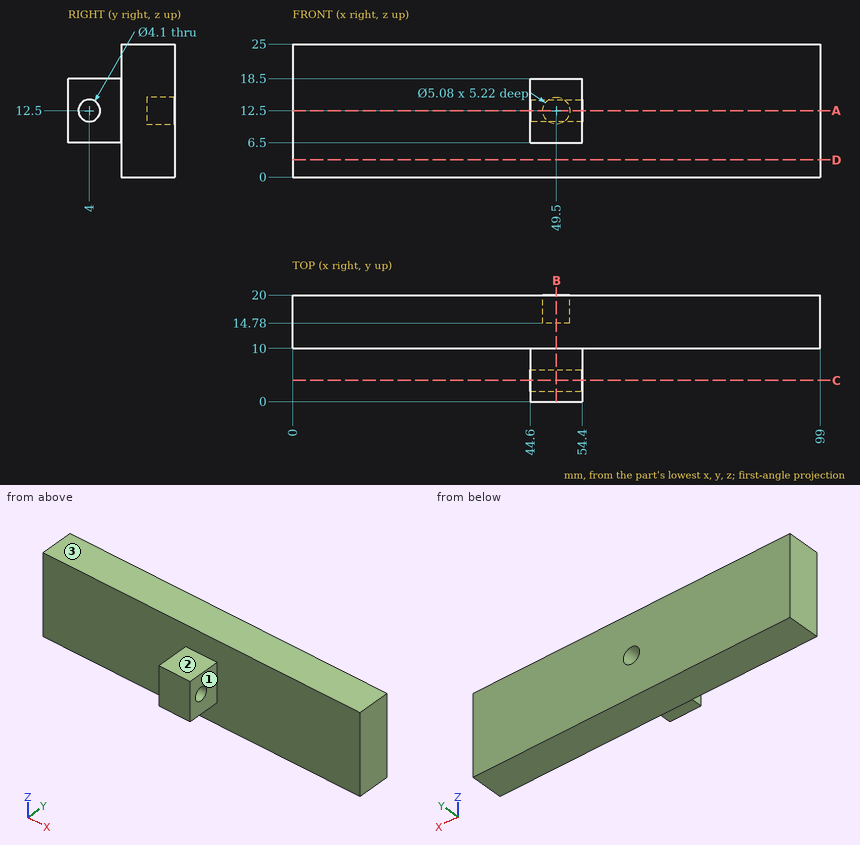
Part print with two shaded views. Sizes in mm from the minimum x, y, z corner. A direction names the side the tool comes from. Round coordinates to 2 decimals unless told otherwise and drop trailing zeros. Write each loop counter-clockwise with the first axis right and the second up, starting at its lowest first coordinate (ties: lowest second). Pieces come first, ordered by that corner, then holes. Notation, with made-up numbers: (5, -4.5) - (51, -4.5) arc R27 cw to (51, 21.5) - close; hole circle Ø2 at (82.25, 86.5). An arc over 180 degrees is marked (long way). Use CSV: the item, a comma, the result in double quotes.
Item 1: Slice it at D-D, the plane z = 3.25. Write the cut outline in (x, y), then the cut area to 3 significant figures.
Results list:
outline,"(0, 10) - (99, 10) - (99, 20) - (0, 20) - close"
area,"990 mm²"
Item 2: Tool access for the marked faces 1, 2 and 3: list every direction of +Z, -Z, +X, -X, +Y, -Y with a clear straight run to the whole face (end or side of a thin tool).
Results list:
face 1,"+Z, -Z, +X, -Y"
face 2,"+Z, +X, -X, -Y"
face 3,"+Z, +X, -X, +Y, -Y"
Item 3: Wall check: L1, parallel to Y at x = 52, z = 12.5; L2, parallel to X at y = 18.25, z = 12.5; L3, parallel to Y at x = 39, z = 15.25. Give the ranges that are in metal, low to high.
Results list:
L1,"y = 0 to 1.95, 6.05 to 14.78"
L2,"x = 0 to 46.96, 52.04 to 99"
L3,"y = 10 to 20"
Item 4: Slice it at A-A, the plane z = 12.5. Write the cut outline in (x, y).
Results list:
outline,"(0, 10) - (44.6, 10) - (44.6, 6.05) - (54.4, 6.05) - (54.4, 10) - (99, 10) - (99, 20) - (52.04, 20) - (52.04, 14.78) - (46.96, 14.78) - (46.96, 20) - (0, 20) - close; (44.6, 0) - (54.4, 0) - (54.4, 1.95) - (44.6, 1.95) - close"
Item 5: Slice it at C-C, the plane y = 4. Write the cut outline in (x, z), then the cut area to 3 significant figures.
Results list:
outline,"(44.6, 6.5) - (54.4, 6.5) - (54.4, 10.45) - (44.6, 10.45) - close; (44.6, 14.55) - (54.4, 14.55) - (54.4, 18.5) - (44.6, 18.5) - close"
area,"77.4 mm²"
Item 6: Flat gauge pins, fed straight in: P1, Ø3, axis at x = 49.5, z = 12.5, coming from the +Y side; P2, Ø11, axis at y = 2.5, z = 13.5, coming from the +X side; P3, Ø3, axis at x = 50, y = 6, coming from the -Z side. Where does each tip first touch, or does it go through?
Results list:
P1,"stops at y = 14.78"
P2,"stops at x = 54.4"
P3,"stops at z = 6.5"
Item 7: Slice it at B-B, the plane x = 49.5. Write the cut outline in (y, z).
Results list:
outline,"(0, 6.5) - (10, 6.5) - (10, 0) - (20, 0) - (20, 9.96) - (14.78, 9.96) - (14.78, 15.04) - (20, 15.04) - (20, 25) - (10, 25) - (10, 18.5) - (0, 18.5) - close; hole circle Ø4.1 at (4, 12.5)"
